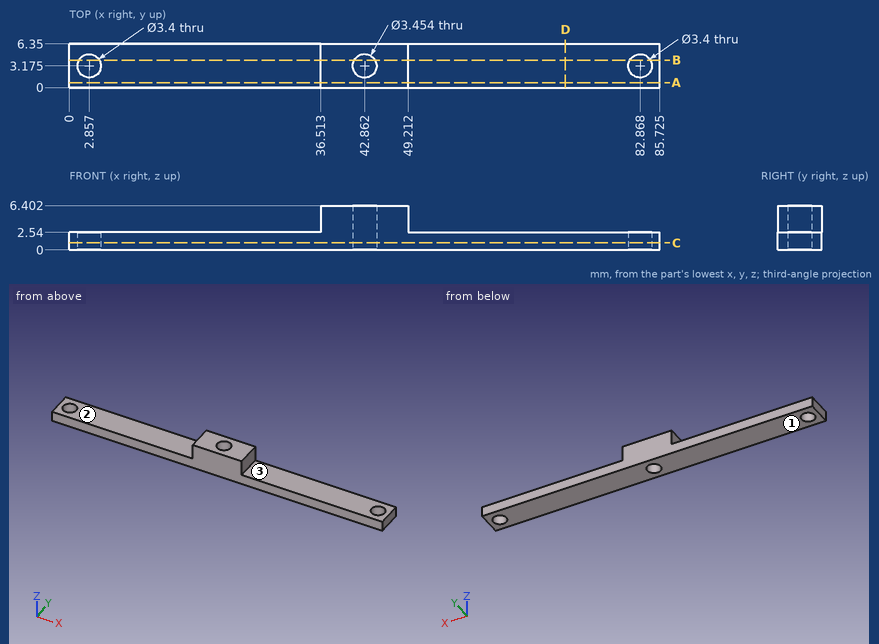
Verification items for this drawing (mm, ordinates from the low corner). A direction names the side the tool comes from. Give positions to 0.01 mm unless a question says otherwise; leave off trailing zeros. Loops run counter-clockwise (first coordinate to the right, second up) from the corner with the lowest first, then second, coordinate; pieces in that order, holes last.
(1) Set-up check for the marked faces 1, 2 and 3: record each of +Z, -Z, +X, -X, +Y, -Y from which the full face is reachable in a straight line by a thin tool's end or side.
From the geometry:
face 1: -Z, +X, -X, +Y, -Y
face 2: +Z, -X, +Y, -Y
face 3: +Z, +X, +Y, -Y
(2) Section check C-C on z = 1. Count the separate pieces of the cut face and the enclosed holes in it, then the cut area to 3 significant figures.
From the geometry:
separate pieces: 1
enclosed holes: 3
area: 517 mm2
(3) Section check B-B on y = 4. Record the cut outline in (x, z) (1 decimal), then the cut area to 3 significant figures.
From the geometry:
outline: (0, 0) - (1.4, 0) - (1.4, 2.5) - (0, 2.5) - close; (4.3, 0) - (41.3, 0) - (41.3, 6.4) - (36.5, 6.4) - (36.5, 2.5) - (4.3, 2.5) - close; (44.4, 0) - (81.4, 0) - (81.4, 2.5) - (49.2, 2.5) - (49.2, 6.4) - (44.4, 6.4) - close; (84.4, 0) - (85.7, 0) - (85.7, 2.5) - (84.4, 2.5) - close
area: 232 mm2
(4) Section check A-A on y = 0.75. Record the cut outline in (x, z) (1 decimal).
From the geometry:
outline: (0, 0) - (85.7, 0) - (85.7, 2.5) - (49.2, 2.5) - (49.2, 6.4) - (36.5, 6.4) - (36.5, 2.5) - (0, 2.5) - close
(5) Section check D-D on x = 72. Record the cut outline in (y, z), then the cut area to 3 significant figures.
From the geometry:
outline: (0, 0) - (6.35, 0) - (6.35, 2.54) - (0, 2.54) - close
area: 16.1 mm2
(6) Depth check by flat-ended pin: pin 1 Ø3 at (x, y) = (11, 3) entering from +Z; pin 2 Ø3 at (y, z) = (2, 4.5) entering from -X; pin 3 Ø1.9 at (y, z) = (3.5, 4.5) entering from +X; pin 4 Ø2 at (x, y) = (42.86, 3.18) entering from +Z. Enter the tip coordinate at first touch or a pass-through.
From the geometry:
pin 1: stops at z = 2.54
pin 2: stops at x = 36.51
pin 3: stops at x = 49.21
pin 4: passes through
(7) Thickness scan on L1, parallel to X at y = 3, z = 1.75 (1 decimal); L2, parallel to X at y = 3.25, z = 1.25 (1 decimal); L3, parallel to X at y = 4, z = 6.25 (1 decimal). Record the ranges inside material, lowest first.
From the geometry:
L1: x = 0 to 1.2, 4.5 to 41.1, 44.6 to 81.2, 84.6 to 85.7
L2: x = 0 to 1.2, 4.6 to 41.1, 44.6 to 81.2, 84.6 to 85.7
L3: x = 36.5 to 41.3, 44.4 to 49.2
